Autodesk Fusion 360 part; units mm, degrees
sketch "Boceto1" plane through (0, 0, 0) normal (0, 0, 1) x (1, 0, 0)
  line L0 (0, 0) -> (46, 0)
  line L1 (46, 0) -> (46, 57)
  line L2 (46, 57) -> (0, 57)
  line L3 (0, 57) -> (0, 0)
  line L4 (-6, 77) -> (52, 77)
  line L5 (52, 77) -> (52, -20)
  line L6 (52, -20) -> (-6, -20)
  line L7 (-6, -20) -> (-6, 77)
  dimension "d1" = 46
  dimension "d2" = 57
  dimension "d3" = 58
  dimension "d4" = 97
  dimension "d5" = 6
  dimension "d6" = 20
extrude "Extruir1" add sketch "Boceto1" against normal blind 2
sketch "Boceto2" plane through (0, 0, -2) normal (0, 0, -1) x (-1, 0, 0)
  line L0 (0, 57) -> (0, 0)
  line L1 (0, 0) -> (-46, 0)
  line L2 (-46, 0) -> (-46, 57)
  line L3 (-46, 57) -> (0, 57)
  line L4 (-52, -20) -> (6, -20)
  line L5 (6, -20) -> (6, 77)
  line L6 (6, 77) -> (-52, 77)
  line L7 (-52, 77) -> (-52, -20)
  line L8 (-46, 57) -> (0, 57)
  line L9 (0, 57) -> (0, 0)
  line L10 (0, 0) -> (-46, 0)
  line L11 (-46, 0) -> (-46, 57)
  line L12 (-49, -17) -> (3, -17)
  line L13 (3, -17) -> (3, 74)
  line L14 (3, 74) -> (-49, 74)
  line L15 (-49, 74) -> (-49, -17)
  circle A0 centre (-25, 65) radius 2.5
  dimension "d9" = -3
  dimension "d10" = 5
extrude "Extruir2" add sketch "Boceto2" along normal blind 14 contours L4 L5 L6 L7
sketch "Boceto3" plane through (0, -17, 0) normal (0, 1, 0) x (-1, 0, 0)
  line L0 (3, -2) -> (-49, -2)
  line L1 (-49, -2) -> (-49, -16)
  line L2 (-49, -16) -> (3, -16)
  line L3 (3, -16) -> (3, -2)
  line L4 (-23, -9) -> (-31, -9)
  ellipse E0 centre (-23, -9) end of major axis (-31, -9) minor radius 4
  line L5 (-15, -9) -> (-31, -9)
  line L6 (-23, -5) -> (-23, -13)
  dimension "d14" = 8
extrude "Extruir3" cut sketch "Boceto3" against normal blind 10 contours L4 E0 L5 L6 | E0 L5 L6 | L4 E0 L5 L6 | E0 L5 L6
extrude "Extruir4" cut sketch "Boceto2" against normal blind 10 contours A0
sketch "Boceto4" plane through (0, 77, 0) normal (0, 1, 0) x (-1, 0, 0)
  line L0 (6, 0) -> (-52, 0)
  line L1 (-52, 0) -> (-52, -16)
  line L2 (-52, -16) -> (6, -16)
  line L3 (6, -16) -> (6, 0)
  line L4 (-52, 0) -> (-52, -16)
  line L5 (-52, 0) -> (-56, 0)
  line L6 (-56, 0) -> (-52, 0)
  line L7 (-52, 0) -> (-52, -4)
  line L8 (-52, -4) -> (-56, -4)
  line L9 (-56, -4) -> (-56, 0)
  line L10 (-52, -4) -> (-52, -8)
  line L11 (-52, -8) -> (-56, -8)
  line L12 (-56, -8) -> (-56, -12)
  line L13 (-56, -12) -> (-52, -12)
  line L14 (-52, -12) -> (-52, -8)
  line L15 (-23, 0) -> (-23, -16)
  line L16 (6, -4) -> (10, -4)
  line L17 (6, 0) -> (10, 0)
  line L18 (10, -4) -> (10, 0)
  line L19 (6, -8) -> (10, -8)
  line L20 (10, -8) -> (10, -12)
  line L21 (10, -12) -> (6, -12)
  dimension "d19" = 4
  dimension "d20" = 4
  dimension "d21" = 4
  dimension "d22" = 4
  dimension "d23" = 4
  dimension "d24" = 4
extrude "Extruir5" add sketch "Boceto4" against normal blind 97 contours L3 L16 L17 L18 | L1 L4 L5 L6 L7 L8 L9 | L3 L19 L20 L21 | L1 L4 L11 L12 L13 L14
sketch "Boceto5" plane through (0, 77, 0) normal (0, 1, 0) x (-1, 0, 0)
  line L0 (10, 0) -> (-56, 0)
  line L1 (-56, 0) -> (-56, -4)
  line L2 (-56, -4) -> (-52, -4)
  line L3 (-52, -4) -> (-52, -8)
  line L4 (-52, -8) -> (-56, -8)
  line L5 (-56, -8) -> (-56, -12)
  line L6 (-56, -12) -> (-52, -12)
  line L7 (-52, -12) -> (-52, -16)
  line L8 (-52, -16) -> (6, -16)
  line L9 (6, -16) -> (6, -12)
  line L10 (6, -12) -> (10, -12)
  line L11 (10, -12) -> (10, -8)
  line L12 (10, -8) -> (6, -8)
  line L13 (6, -8) -> (6, -4)
  line L14 (6, -4) -> (10, -4)
  line L15 (10, -4) -> (10, 0)
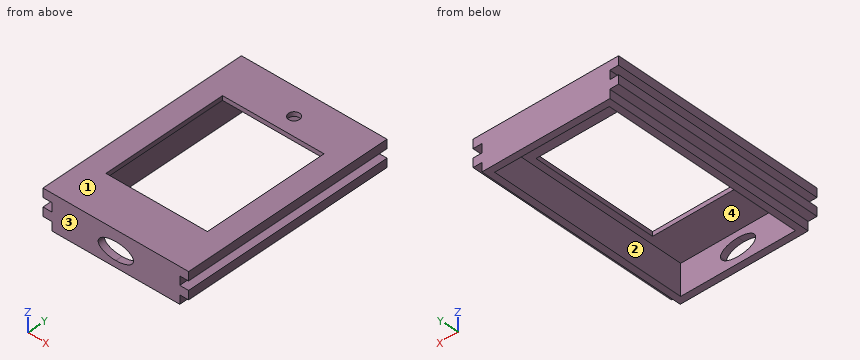
Here's how the part is built. I have some questions about the finished solid (model axes, mm). Face numbers are marked on the shaded views. A direction names the side the tool comes from. Give positions to 0.01 mm unless a question says otherwise; leave off trailing zeros. Order: outer loops, then holes, each group sorted by start corner. A loop starts at its lowest first (then second) coordinate and runs counter-clockwise, first axis right, second up. Notation, with made-up numbers: (32.25, -3.5) -> (41.25, -3.5) arc R24 cw to (41.25, 28.5) -> close; hole circle Ø6 at (-35.75, 31.25). An arc over 180 degrees is marked (long way). One line per item, written item: value. Start each with the question number.
1. Imagine slicing it at D-D, the plane x = 25. Count the separate pieces of the cut face and the enclosed holes in it, plus the area to 3 significant figures.
2. We'd pull the mould along X, two halves only. Please class the marked faces 1 and 2: released by +X, released by -X, zero draft, split by the parting line, or undercut.
3. Imagine slicing it at B-B, the plane y = 65. List the corners of the cut face in (x, z) for me.
4. Will these pins go through, and if not, where does the flat tip stop? pin 1 Ø1.2 at (y, z) = (50.5, -7) entering from +X; pin 2 Ø2 at (y, z) = (9.5, -14.5) entering from -X; pin 3 Ø1.2 at (x, y) = (54, 40) entering from -Z.
5. Imagine slicing it at A-A, the plane z = -14.75. List the corners of the cut face in (x, y) for me, plus the area to 3 significant figures.
6. Imagine slicing it at C-C, the plane y = 10.5. List the corners of the cut face in (x, z) for me.
7. For the marked faces 3 and 4, which set-ups out of +Z, -Z, +X, -X, +Y, -Y let a thin tool reach every point of the face, with its end or its side?
8. I need wall thicknesses on probe 1 along Y at (x, z) = (17, -6); probe 2 along Y at (x, z) = (32.5, -0.75); probe 3 along X at (y, z) = (37.5, -2.25). Which ranges of each line are inside material? Lowest first, please. Write a range as from..to.
Values follow:
1. separate pieces: 4
1. enclosed holes: 0
1. area: 131 mm2
2. face 1: zero draft
2. face 2: undercut
3. outline: (-10, -12) -> (-6, -12) -> (-6, -16) -> (-3, -16) -> (-3, -2) -> (22.5, -2) -> (22.5, 0) -> (-10, 0) -> (-10, -4) -> (-6, -4) -> (-6, -8) -> (-10, -8) -> close; (27.5, -2) -> (49, -2) -> (49, -16) -> (52, -16) -> (52, -12) -> (56, -12) -> (56, -8) -> (52, -8) -> (52, -4) -> (56, -4) -> (56, 0) -> (27.5, 0) -> close
4. pin 1: stops at x = 52
4. pin 2: stops at x = -6
4. pin 3: stops at z = -12
5. outline: (-6, -20) -> (52, -20) -> (52, 77) -> (-6, 77) -> close; hole (-3, -17) -> (49, -17) -> (49, 74) -> (-3, 74) -> close
5. area: 894 mm2
6. outline: (-10, -12) -> (-6, -12) -> (-6, -16) -> (-3, -16) -> (-3, -2) -> (0, -2) -> (0, 0) -> (-10, 0) -> (-10, -4) -> (-6, -4) -> (-6, -8) -> (-10, -8) -> close; (46, -2) -> (49, -2) -> (49, -16) -> (52, -16) -> (52, -12) -> (56, -12) -> (56, -8) -> (52, -8) -> (52, -4) -> (56, -4) -> (56, 0) -> (46, 0) -> close
7. face 3: +Z, -Z, +X, -X, -Y
7. face 4: -Z
8. probe 1: y = -20..-17, 74..77
8. probe 2: y = -20..0, 57..77
8. probe 3: x = -10..-3, 49..56
